Autodesk Inventor part; units mm, degrees
ref_plane "YZ Plane" through (0, 0, 0) normal (1, 0, 0) x (0, 1, 0)
ref_plane "XZ Plane" through (0, 0, 0) normal (0, 1, 0) x (-1, 0, 0)
ref_plane "XY Plane" through (0, 0, 0) normal (0, 0, 1) x (1, 0, 0)
sketch "Sketch1" plane through (0, 0, 0) normal (0, 1, 0) x (-1, 0, 0)
  line L0 (200.025, 436.88) -> (-200.025, 436.88)
  line L1 (-200.025, 436.88) -> (-200.025, -436.88)
  line L2 (-200.025, -436.88) -> (200.025, -436.88)
  line L3 (200.025, -436.88) -> (200.025, 436.88)
  line L4 (200.025, 436.88) -> (-200.025, -436.88) construction
  line L5 (-200.025, 436.88) -> (200.025, -436.88) construction
  point P0 (0, 0)
  dimension "d0" = 400.05
  dimension "d1" = 873.76
extrude "Extrusion1" add sketch "Sketch1" along normal blind 12.7
sketch "Sketch4" plane through (0, 12.7, 0) normal (0, 1, 0) x (1, 0, 0)
  line L0 (-82.55, -436.88) -> (82.55, -436.88)
  line L1 (82.55, -436.88) -> (82.55, -233.68)
  line L2 (82.55, -233.68) -> (-82.55, -233.68)
  line L3 (-82.55, -233.68) -> (-82.55, -436.88)
  line L4 (-82.55, -436.88) -> (82.55, -233.68) construction
  line L5 (82.55, -436.88) -> (-82.55, -233.68) construction
  line L6 (-200.025, -436.88) -> (200.025, -436.88)
  line L7 (-200.025, 436.88) -> (-200.025, -436.88)
  line L8 (200.025, -436.88) -> (200.025, 436.88)
  point P0 (0, 0)
  point P1 (0, -335.28)
  dimension "d11" = 0
  dimension "d12" = 165.1
  dimension "d13" = 203.2
  dimension "d19" = 117.475
  dimension "d20" = 117.475
extrude "Extrusion2" cut sketch "Sketch4" against normal through all
sketch "Sketch6" plane through (0, 12.7, 0) normal (0, 1, 0) x (1, 0, 0)
  line L0 (0, 0) -> (0, -436.88) construction
  line L1 (-104.775, -360.68) -> (104.775, -360.68)
  line L2 (104.775, -360.68) -> (104.775, -436.88)
  line L3 (104.775, -436.88) -> (-104.775, -436.88)
  line L4 (-104.775, -436.88) -> (-104.775, -360.68)
  line L5 (-104.775, -360.68) -> (104.775, -436.88) construction
  line L6 (104.775, -360.68) -> (-104.775, -436.88) construction
  line L7 (-200.025, -436.88) -> (-82.55, -436.88)
  point P0 (0, -398.78)
  dimension "d24" = 209.55
  dimension "d25" = 76.2
extrude "Extrusion4" cut sketch "Sketch6" against normal through all
properties part number "2020 Wood Base" material "Wood (Birch)"
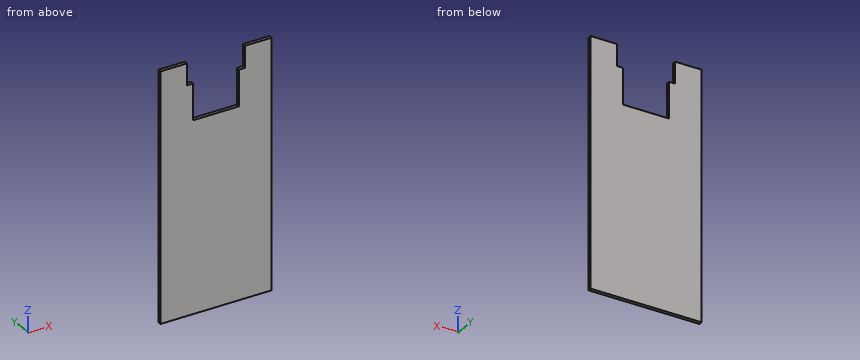
Read the model definition and answer for the solid it produces. Units are mm, in the model's axes. Give positions to 0.01 mm unless a question says otherwise; leave off trailing zeros. Loops run counter-clockwise (first coordinate to the right, second up) from the corner with the lowest first, then second, coordinate; pieces in that order, holes last.
Item 1: Each of these flat-tipped pins is pushed along its axis until it touches: pin 1 Ø4 at (x, y) = (-6.5, 5) entering from +Z; pin 2 Ø6.5 at (x, y) = (-92, 8) entering from +Z. Where does it stop, or does it pass through?
Item 2: The part is cut by section B-B (x = 67). Write down the section's boundary in (y, z), and give its area (3 significant figures).
Item 3: The part is cut by section A-A (y = 8). Write down the section's boundary in (x, z) (3 decimals).
Item 4: Find the intervals of material crossed by line 1 along Z through (x, y) = (-67.5, 1); line 2 along Z through (x, y) = (97, 6.75), in increasing order.
Taken from the geometry:
1. pin 1: stops at z = 233.68
1. pin 2: stops at z = 360.68
2. outline: (0, -436.88) - (12.7, -436.88) - (12.7, 233.68) - (0, 233.68) - close
2. area: 8,520 mm2
3. outline: (-200.025, -436.88) - (200.025, -436.88) - (200.025, 436.88) - (104.775, 436.88) - (104.775, 360.68) - (82.55, 360.68) - (82.55, 233.68) - (-82.55, 233.68) - (-82.55, 360.68) - (-104.775, 360.68) - (-104.775, 436.88) - (-200.025, 436.88) - close
4. line 1: z = -436.88 to 233.68
4. line 2: z = -436.88 to 360.68
